Can you work these out from the model? Positions are in its coordinate system, mm. A direction names the side the tool comes from. Coordinates: 2 decimals unless noted, no trailing zeros. Order: outer loops, then holes, each group sorted by start corner. A loop starts at its lowest first (then second) coordinate and runs counter-clockwise, first axis right, second up. Notation, with made-up numbers: (21, 40) -> (69, 40) arc R24 ccw to (69, 56) -> close; hole circle Ø2 at (-15.5, 56). An arc over 180 degrees is marked (long way). Answer as a JSON object with one key per item and string values. Group by question number.
(1) Which directions (+Z, -Z, +X, -X, +Y, -Y) give clear straight access to the entire face, cutting with the end or side of a thin tool? Please do faces 1 (the flat face through (-21, 20.5, 10)), 2 (the flat face through (77, 15, 10)), 3 (the flat face through (82, 20, 10)).
(2) For pin 1 (10.5 mm diameter, centred on x = -5.5, z = 14.5, fed in from -Y); pin 2 (1.5 mm diameter, centred on x = -20.5, z = 5, fed in from -Y); pin 3 (3 mm diameter, centred on y = 13, z = 7.5, fed in from -X), each with a flat end and sliding along its axis, tell me the tip position at first contact or that it passes through.
(3) I want a section at B-B, the plane z = 3.5. List the corners of the cut face in (x, y) for me, plus the area to 3 significant figures.
(4) I want a section at D-D, the plane x = 54. List the corners of the cut face in (y, z) for me.
(5) I want a section at A-A, the plane y = 13. List the corners of the cut face in (x, z) for me, plus the area to 3 significant figures.
(6) I need wall thicknesses on line 1 (Y direction, x = 3.2, z = 10); line 2 (X direction, y = 45, z = 3); line 3 (Y direction, x = 23.5, z = 6). Which ranges of each line are inside material? Lowest first, please.
(7) If we mould it in two halves opening along Z, with no side actions, what happens to faces 4 (the conical face through (6.479, 73.252, 10.112)), 5 (the flat face through (40, 0, 10)), 6 (the flat face through (8, 42, 20))? For each: pulls with the +Z half, pulls with the -Z half, needs draft (parallel to the pull), parting line crosses it, or undercut.
(8) I want a section at C-C, the plane y = 29. List the corners of the cut face in (x, z) for me.
from build123d import *

# Parameters (mm, degrees)
F1_DEPTH       = 20
F2_R           = 5
F3_R           = 5
F4_R           = 5
F6_D           = 4
F6_CSINK_D     = 8
F6_CSINK_ANGLE = 45


with BuildPart() as f1:
    # F0 (on Top) → F1 (new body)
    with BuildSketch(Plane.XY):
        Polygon((0, 80.5), (0, 0), (87, 0), (87, 20), (77, 20), (77, 10), (10, 10), (10, 90.5), (-28, 90.5), (-28, 20.5), (-13, 20.5), (-13, 80.5), align=None)
    extrude(amount=F1_DEPTH)

    # F2
    f2_edges = [f1.edges().sort_by_distance(p)[0] for p in [
        (87, 0, 10),
    ]]
    fillet(f2_edges, radius=F2_R)

    # F3
    f3_edges = [f1.edges().sort_by_distance(p)[0] for p in [
        (-13, 20.5, 10),
        (-28, 20.5, 10),
    ]]
    fillet(f3_edges, radius=F3_R)

    # F4
    f4_edges = [f1.edges().sort_by_distance(p)[0] for p in [
        (-28, 90.5, 10),
        (10, 90.5, 10),
    ]]
    fillet(f4_edges, radius=F4_R)

    # F6 (through all)
    with Locations(Plane.YZ.offset(10)):
        with Locations((70.712887, 10), (44.433817, 10)):
            CounterSinkHole(F6_D / 2, F6_CSINK_D / 2, counter_sink_angle=F6_CSINK_ANGLE)


solid = f1.part
Computed values:
{
 "1": {"face 1": "+Z, -Z, -X, -Y", "face 2": "+Z, -Z, +Y", "face 3": "+Z, -Z, +X, +Y"},
 "2": {"pin 1": "stops at y = 80.5", "pin 2": "stops at y = 20.5", "pin 3": "stops at x = 0"},
 "3": {"outline": "(-28, 25.5) arc R5 ccw to (-23, 20.5) -> (-18, 20.5) arc R5 ccw to (-13, 25.5) -> (-13, 80.5) -> (0, 80.5) -> (0, 0) -> (82, 0) arc R5 ccw to (87, 5) -> (87, 20) -> (77, 20) -> (77, 10) -> (10, 10) -> (10, 85.5) arc R5 ccw to (5, 90.5) -> (-23, 90.5) arc R5 ccw to (-28, 85.5) -> close", "area": "2,930 mm2"},
 "4": {"outline": "(0, 0) -> (10, 0) -> (10, 20) -> (0, 20) -> close"},
 "5": {"outline": "(0, 0) -> (10, 0) -> (10, 20) -> (0, 20) -> close; (77, 0) -> (87, 0) -> (87, 20) -> (77, 20) -> close", "area": "400 mm2"},
 "6": {"line 1": "y = 0 to 42.43, 46.43 to 68.71, 72.71 to 90.5", "line 2": "x = -28 to -13, 0 to 10", "line 3": "y = 0 to 10"},
 "7": {"face 4": "undercut", "face 5": "needs draft", "face 6": "pulls with the +Z half"},
 "8": {"outline": "(-28, 0) -> (-13, 0) -> (-13, 20) -> (-28, 20) -> close; (0, 0) -> (10, 0) -> (10, 20) -> (0, 20) -> close"}
}
